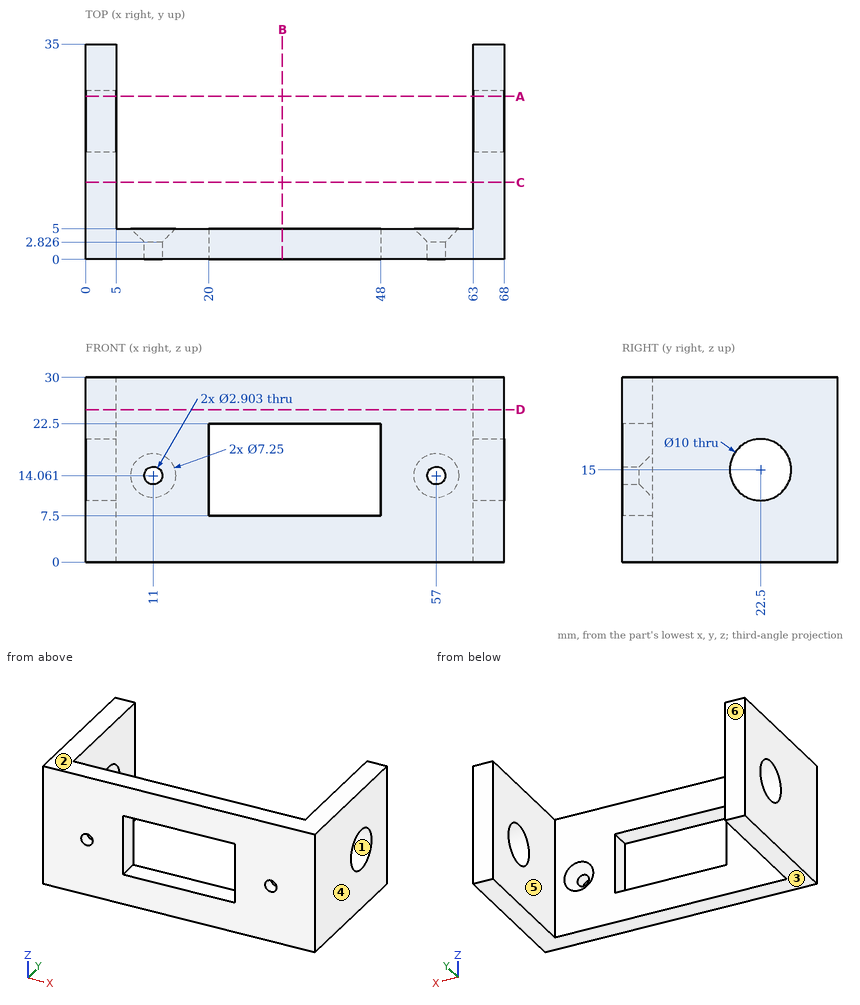
The drawing under review shows one solid part. Ordinate dimensions are in mm from its lowest x, y, z. A direction names the side the tool comes from. Coordinates: 2 decimals unless noted, no trailing zeros. Order: outer loops, then holes, each group sorted by start corner. A loop starts at its lowest first (then second) coordinate and runs counter-clockwise, first axis right, second up. Notation, with made-up numbers: (59.5, 77.5) -> (99.5, 77.5) arc R29 cw to (99.5, 99.5) -> close; hole circle Ø10 at (31.25, -25). An arc over 180 degrees is marked (long way). One line per item, written item: value.
1) We need section D-D, the plane z = 24.75. Give the boundary of the cut face in (x, y).
Output values:
outline: (0, 0) -> (68, 0) -> (68, 35) -> (63, 35) -> (63, 5) -> (5, 5) -> (5, 35) -> (0, 35) -> close
2) To check wall thickness, follow probe 1 along X at (y, z) = (15.5, 23.5); probe 2 along Y at (x, z) = (64.65, 15); probe 3 along Z at (x, y) = (11, 1.3). State the ranges of each line that lie inside material, in increasing order. Write a range as [from, to].
Output values:
probe 1: x = [0, 5], [63, 68]
probe 2: y = [0, 17.5], [27.5, 35]
probe 3: z = [0, 12.61], [15.51, 30]
3) We need section A-A, the plane y = 26.5. Give the boundary of the cut face in (x, z).
Output values:
outline: (0, 0) -> (5, 0) -> (5, 12) -> (0, 12) -> close; (0, 18) -> (5, 18) -> (5, 30) -> (0, 30) -> close; (63, 0) -> (68, 0) -> (68, 12) -> (63, 12) -> close; (63, 18) -> (68, 18) -> (68, 30) -> (63, 30) -> close
4) Draft analysis for pull direction Z (two halves, no side actions). For the marked faces 1, 2, 3 and 4, state which applies: +Z half, -Z half, draft (parallel to the pull), parting line (faces both ways), or undercut.
Output values:
face 1: undercut
face 2: +Z half
face 3: -Z half
face 4: draft
5) Clearance check with flat-ended pins moving along their axes: P1, Ø10, axis at x = 9, y = 12.5, coming from the -Z side; P2, Ø9, axis at x = 47.5, z = 11, coming from the +Y side; P3, Ø2, axis at x = 57, z = 13.5, coming from the +Y side (1 decimal). State where each tip first meets the part, or that it passes through.
Output values:
P1: stops at z = 0
P2: stops at y = 5
P3: stops at y = 2.9
6) We need section C-C, the plane y = 12.5. Give the boundary of the cut face in (x, z), then the cut area to 3 significant figures.
Output values:
outline: (0, 0) -> (5, 0) -> (5, 30) -> (0, 30) -> close; (63, 0) -> (68, 0) -> (68, 30) -> (63, 30) -> close
area: 300 mm2
7) Machinability: for the marked faces 5 and 6, which of the approach directions +Z, -Z, +X, -X, +Y, -Y give a long, thin tool a straight path to every point of the face, cutting with its end or side? Answer none if there is none.
Output values:
face 5: +Z, -Z, +Y
face 6: +Z, -Z, +X, -X, +Y
8) We need section B-B, the plane x = 32. Give the boundary of the cut face in (y, z).
Output values:
outline: (0, 0) -> (5, 0) -> (5, 7.5) -> (0, 7.5) -> close; (0, 22.5) -> (5, 22.5) -> (5, 30) -> (0, 30) -> close
